from build123d import *

# Parameters (mm, degrees)
CUT_EXTRUDE1_START       = -5
CUT_EXTRUDE1_DEPTH       = 5
FILLET1_R                = 1.5
CHAMFER1_SIZE            = 5
CIRPATTERN2_COUNT        = 3
FILLET1_OF_CIRPATTERN2_R = 1.5
CIRPATTERN3_COUNT        = 6


with BuildPart() as part:
    # Sketch2 → Revolve1 (revolve)
    with BuildSketch(Plane(origin=(0, 0, 0), x_dir=(0, 0, -1), z_dir=(1, 0, 0)), mode=Mode.PRIVATE) as revolve1_sk:
        Polygon((-55, 0), (-80, 0), (-80, 15), (-65, 15), (-65, 10), (-55, 10), align=None)
    revolve(revolve1_sk.sketch.rotate(Axis((0, -0.75, 0), (0, 1, 0)), 180), axis=Axis((0, -0.75, 0), (0, 1, 0)))

    # Sketch4 → Cut-Extrude1 (cut)
    with BuildSketch(Plane(origin=(0, 15, 0), x_dir=(1, 0, 0), z_dir=(0, 1, 0)).offset(CUT_EXTRUDE1_START)):
        with BuildLine():
            Line((-3.881158746, 64.88402428), (-8.835527397, 71.959595994))
            ThreePointArc((-8.835527397, 71.959595994), (0, 72.5), (8.835527397, 71.959595994))
            Line((8.835527397, 71.959595994), (3.881158746, 64.88402428))
            ThreePointArc((3.881158746, 64.88402428), (0, 65), (-3.881158746, 64.88402428))
        make_face()
    cut_extrude1 = extrude(amount=CUT_EXTRUDE1_DEPTH, mode=Mode.SUBTRACT)

    # Fillet1
    fillet1_edges = [part.edges().sort_by_distance(p)[0] for p in [
        (3.881158746, 12.5, -64.88402428),
        (-3.881158746, 12.5, -64.88402428),
        (-8.835527397, 12.5, -71.959595994),
        (8.835527397, 12.5, -71.959595994),
    ]]
    fillet(fillet1_edges, radius=FILLET1_R)

    # Chamfer1
    chamfer1_edges = [part.edges().sort_by_distance(p)[0] for p in [
        (0, 0, 55),
    ]]
    chamfer(chamfer1_edges, length=CHAMFER1_SIZE)

    # CirPattern2: Cut-Extrude1 ×3 about axis
    cirpattern2_axis = Axis((0, 0, 0), (0, 1, 0))
    for i in range(1, CIRPATTERN2_COUNT):
        add(cut_extrude1.rotate(cirpattern2_axis, i * 360 / CIRPATTERN2_COUNT), mode=Mode.SUBTRACT)

    # Fillet1 of CirPattern2
    fillet1_of_cirpattern2_edges = [part.edges().sort_by_distance(p)[0] for p in [
        (-58.131792699, 12.5, 29.08083007),
        (-54.250633954, 12.5, 35.80319421),
        (-57.901074478, 12.5, 43.631589179),
        (-66.736601875, 12.5, 28.328006815),
        (54.250633954, 12.5, 35.80319421),
        (58.131792699, 12.5, 29.08083007),
        (66.736601875, 12.5, 28.328006815),
        (57.901074478, 12.5, 43.631589179),
    ]]
    fillet(fillet1_of_cirpattern2_edges, radius=FILLET1_OF_CIRPATTERN2_R)

    # Sketch7 → #10-32 Tapped Hole1 (revolve, cut)
    with BuildSketch(Plane(origin=(-36.25, 15, -62.786841774), x_dir=(0, 0, 1), z_dir=(1, 0, 0))):
        Polygon((0, 0), (0, 11.213317848), (2.0193, 10), (2.0193, 0), align=None)
    f_10_32_tapped_hole1 = revolve(axis=Axis((-36.25, 21.35, -62.786841774), (0, -1, 0)), mode=Mode.SUBTRACT)

    # CirPattern3: #10-32 Tapped Hole1 ×6 about axis
    cirpattern3_axis = Axis((0, 0, 0), (0, 1, 0))
    for i in range(1, CIRPATTERN3_COUNT):
        add(f_10_32_tapped_hole1.rotate(cirpattern3_axis, i * 360 / CIRPATTERN3_COUNT), mode=Mode.SUBTRACT)


solid = part.part
Check sheet for the modelled part. Datum: model origin and axes. Units: mm. A direction names the side the tool comes from. Round coordinates to 2 decimals unless told otherwise and drop trailing zeros. Loops run counter-clockwise (first coordinate to the right, second up) from the corner with the lowest first, then second, coordinate; pieces in that order, holes last. Notation, with made-up numbers: M 77.25,86.5 L 135.25,86.5 A9 cw 135.25,96.5 Z; hole C 24,-12 d11. An arc over 180 degrees is marked long. One line per question, with ' | ' between items. Start each with the question number.
Item 1: Gauge pin test, flat ends, axial feed: pin 1 Ø2 at (y, z) = (11, -43) entering from +X; pin 2 Ø6 at (x, y) = (31, 9) entering from -Z; pin 3 Ø5 at (y, z) = (12.5, 18.5) entering from +X. Record the tip position at first contact, or that the pin passes through.
Item 2: Release check for a two-part mould opening along Z. For faces 3 (the face through (-60, 0, 11)), 4 (the face through (-62.5, 12.5, 28.7)), 5 (the face through (-3.517, 7.605, 79.923)) record: released by +Z, released by -Z, zero draft, split by the parting line, or undercut.
Item 3: Section check A-A (x = 0). Record the boundary of the cut face in (y, z), and give its area (4 significant figures).
Item 4: Set-up check for faces 1 (the face through (48.794, 7.465, -25.379)), 2 (the face through (48.5, 10, 27.1)): record each of +Z, -Z, +X, -X, +Y, -Y from which the full face is reachable in a straight line by a thin tool's end or side.
Item 5: Scan lines: probe 1 along X at (y, z) = (8, 0); probe 2 along X at (y, z) = (12.5, 0); probe 3 along Z at (x, y) = (34.5, 13.25). Record each from-to range of solid material in increasing order.
Worked out:
1) pin 1: x = 68.09 | pin 2: z = -74.94 | pin 3: x = 78.38
2) face 3: zero draft | face 4: undercut | face 5: split by the parting line
3) outline: M 0,-80 L 15,-80 L 15,-72.5 L 10,-72.5 L 10,-55 L 5,-55 L 0,-60 Z; M 0,60 L 5,55 L 10,55 L 10,65 L 15,65 L 15,80 L 0,80 Z | area: 587.5 mm^2
4) face 1: +Y, -Y | face 2: +Y
5) probe 1: -80 to -74.52, -70.48 to -55, 55 to 70.48, 74.52 to 80 | probe 2: -80 to -74.52, -70.48 to -65, 65 to 70.48, 74.52 to 80 | probe 3: -72.18 to -63.79, -61.78 to -55.09, 55.09 to 61.78, 63.79 to 72.18
